The drawing under review shows one solid part. Ordinate dimensions are in mm from its lowest x, y, z. A direction names the side the tool comes from. Give positions to 0.01 mm unless a question says otherwise; leave off trailing zeros. Order: outer loops, then holes, each group sorted by start corner. A loop starts at its lowest first (then second) coordinate and runs counter-clockwise, first axis right, second up. Notation, with made-up numbers: (72, -24.5) - (124, -24.5) arc R13 ccw to (124, -14.5) - close; hole circle Ø5 at (-13.75, 40). An arc over 180 degrees is marked (long way). Write item = value, one per line. Start each with the question number.
1. Wall thickness on probe 1 along Y at (x, z) = (4, 1); probe 2 along Y at (x, z) = (5, 8.75); probe 3 along Z at (x, y) = (3.75, 1.75): over which ranges is each line inside the solid? List them lowest first.
2. For P1, Ø5, axis at x = 6.5, y = 5.5, coming from the -Z side; P2, Ø0.8, axis at y = 17.5, z = 5, coming from the +X side; P3, Ø2, axis at x = 7, z = 7.5, coming from the +Y side, all flat-tipped, find the tip position at first contact; note any pin that passes through.
3. We need section A-A, the plane y = 14.75. Give the boundary of the cut face in (x, z).
4. We need section B-B, the plane y = 10.5. Give the boundary of the cut face in (x, z).
5. Machinability: for the marked faces 1, 2 and 3, which of the approach directions +Z, -Z, +X, -X, +Y, -Y give a long, thin tool a straight path to every point of the face, cutting with its end or side? Answer none if there is none.
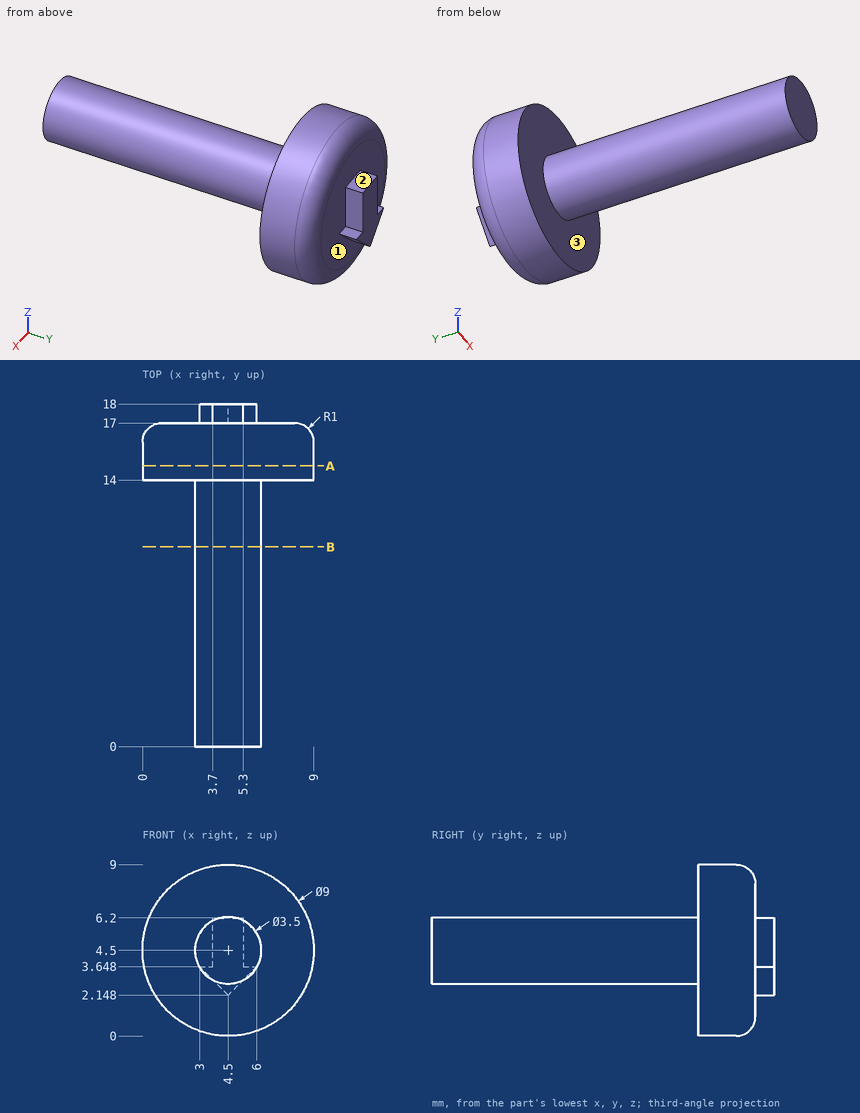
Model answer:
q1.probe_1 = 14 to 17
q1.probe_2 = 14 to 16.63
q1.probe_3 = 2.92 to 6.08
q2.P1 = 2.75
q2.P2 = 5.3
q2.P3 = 17
q3.outline = circle Ø9 at (4.5, 4.5)
q4.outline = circle Ø3.5 at (4.5, 4.5)
q5.face_1 = +Y
q5.face_2 = +Z, +X, -X, +Y
q5.face_3 = -Y
